The listing builds one solid part. Answer for the finished solid, in the listing's coordinates (mm). Face numbers are marked on the shaded views. A direction names the side the tool comes from. Give positions to 0.01 mm unless a question says otherwise; leave off trailing zeros. Order: outer loops, then holes, each group sorted by start corner. A loop starts at its lowest first (then second) coordinate and runs counter-clockwise, first axis right, second up. Notation, with made-up numbers: (-7.75, 33.25) -> (18.25, 33.25) arc R24 cw to (18.25, 69.25) -> close; hole circle Ø6 at (35, -10). An arc over 180 degrees is marked (long way). One line per question, with ' | ' between items. Start each with the question number.
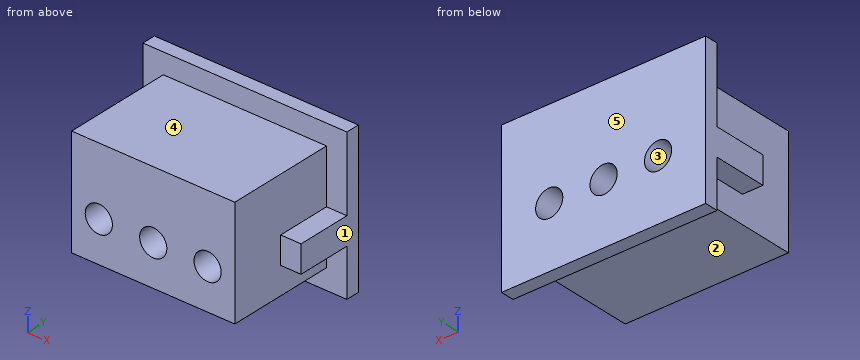
```python
from build123d import *

# Parameters (mm, degrees)
SKETCH1_W           = 6
SKETCH1_H           = 4
BOSS_EXTRUDE1_DEPTH = 4
SKETCH2_W           = 1
SKETCH2_H           = 2
BOSS_EXTRUDE2_DEPTH = 0.75
SKETCH3_W           = 7.5
SKETCH3_H           = 5.5
BOSS_EXTRUDE3_DEPTH = 0.5
SKETCH4_R           = 0.5
CUT_EXTRUDE1_DEPTH  = 7.471089553


with BuildPart() as part:
    # Sketch1 → Boss-Extrude1 (new body)
    with BuildSketch(Plane(origin=(0, 0, 0), x_dir=(1, 0, 0), z_dir=(0, 1, 0))):
        Rectangle(SKETCH1_W, SKETCH1_H)
    extrude(amount=BOSS_EXTRUDE1_DEPTH)

    # Sketch2 → Boss-Extrude2 (add)
    with BuildSketch(Plane(origin=(3, 0, 0), x_dir=(0, 0, -1), z_dir=(1, 0, 0))):
        with Locations((0.5, 3)):
            Rectangle(SKETCH2_W, SKETCH2_H)
    boss_extrude2 = extrude(amount=BOSS_EXTRUDE2_DEPTH)

    # Mirror1: Boss-Extrude2 across plane
    add(boss_extrude2.mirror(Plane(origin=(0, 0, 0), x_dir=(0, 0, 1), z_dir=(1, 0, 0))))

    # Sketch3 → Boss-Extrude3 (add)
    with BuildSketch(Plane(origin=(0, 4, 0), x_dir=(1, 0, 0), z_dir=(0, 1, 0))):
        Rectangle(SKETCH3_W, SKETCH3_H)
    extrude(amount=BOSS_EXTRUDE3_DEPTH)

    # Sketch4 → Cut-Extrude1 (cut, through all)
    with BuildSketch(Plane.XZ):
        with Locations(Location((-2, -0.5, 0), (0, 0, 270))):
            Circle(SKETCH4_R)
        with Locations(Location((0, -0.5, 0), (0, 0, 270))):
            Circle(SKETCH4_R)
        with Locations(Location((2, -0.5, 0), (0, 0, 270))):
            Circle(SKETCH4_R)
    extrude(amount=-CUT_EXTRUDE1_DEPTH, mode=Mode.SUBTRACT)


solid = part.part
```
(1) Consider line 1 (X direction, y = 3.35, z = -0.5); line 2 (X direction, y = 1.95, z = -0.5); line 3 (X direction, y = 3.75, z = -1.9). Determine where each line is inside the solid, lowest interval first.
(2) The part is cut by section D-D on z = 0.35. Determine the outline of the cut face in (x, y).
(3) Determine the mould class of the marked faces 3, 4 and 5 for opening direction Z: pulls with the +Z half, pulls with the -Z half, needs draft (parallel to the pull), parting line crosses it, or undercut.
(4) The part is cut by section B-B on x = 0. Determine the outline of the cut face in (y, z).
(5) Given P1, Ø0.6, axis at x = -3.5, y = 3.5, coming from the -Z side; P2, Ø2, axis at x = 1, y = 1.5, coming from the -Z side; P3, Ø1.2, axis at x = 0, y = 2, coming from the +Z side, each flat-ended and moving along its own axis, determine where each tip first touches the part or whether it passes through.
(6) For the marked faces 1 and 2, determine the directions among +Z, -Z, +X, -X, +Y, -Y from which every point of the face is accessible in a straight line to the end or side of a thin tool.
(7) The part is cut by section A-A on z = -0.5. Determine the outline of the cut face in (x, y).
(8) The part is cut by section C-C on y = 3.45. Determine the outline of the cut face in (x, z), plus the area to 3 significant figures.
Result sheet:
1) line 1: x = -3.75 to -2.5, -1.5 to -0.5, 0.5 to 1.5, 2.5 to 3.75 | line 2: x = -3 to -2.5, -1.5 to -0.5, 0.5 to 1.5, 2.5 to 3 | line 3: x = -3 to 3
2) outline: (-3.75, 4) -> (-3, 4) -> (-3, 0) -> (3, 0) -> (3, 4) -> (3.75, 4) -> (3.75, 4.5) -> (-3.75, 4.5) -> close
3) face 3: undercut | face 4: pulls with the +Z half | face 5: needs draft
4) outline: (0, -2) -> (4, -2) -> (4, -2.75) -> (4.5, -2.75) -> (4.5, -1) -> (0, -1) -> close; (0, 0) -> (4.5, 0) -> (4.5, 2.75) -> (4, 2.75) -> (4, 2) -> (0, 2) -> close
5) P1: stops at z = -1 | P2: stops at z = -2 | P3: stops at z = 2
6) face 1: +Z, -Z, +X, +Y, -Y | face 2: -Z, +X, -X, -Y
7) outline: (-3.75, 2) -> (-3, 2) -> (-3, 0) -> (-2.5, 0) -> (-2.5, 4.5) -> (-3.75, 4.5) -> close; (-1.5, 0) -> (-0.5, 0) -> (-0.5, 4.5) -> (-1.5, 4.5) -> close; (0.5, 0) -> (1.5, 0) -> (1.5, 4.5) -> (0.5, 4.5) -> close; (2.5, 0) -> (3, 0) -> (3, 2) -> (3.75, 2) -> (3.75, 4.5) -> (2.5, 4.5) -> close
8) outline: (-3.75, -1) -> (-3, -1) -> (-3, -2) -> (3, -2) -> (3, -1) -> (3.75, -1) -> (3.75, 0) -> (3, 0) -> (3, 2) -> (-3, 2) -> (-3, 0) -> (-3.75, 0) -> close; hole circle Ø1 at (-2, -0.5); hole circle Ø1 at (0, -0.5); hole circle Ø1 at (2, -0.5) | area: 23.1 mm^2
